Source: three-view drawing plus pictorial views. Frame: mm from the lowest corner of the part. A direction names the side the tool comes from. Round coordinates to 2 decimals unless told otherwise and drop trailing zeros. Order: outer loops, then holes, each group sorted by start corner. A loop starts at its lowest first (then second) coordinate and runs counter-clockwise, first axis right, second up. Notation, with made-up numbers: M 2.25,87.25 L 54.25,87.25 A29 ccw 54.25,120.25 Z; hole C -23,-14 d3. An arc over 180 degrees is marked long. Return JSON: item names as keys, results as strings. Group by question number.
Q1. Ray query, probe 1 along Y at (x, z) = (3.95, 10.5); probe 2 along Z at (x, y) = (5.35, 2.5); probe 3 along Z at (x, y) = (4.8, 9.75). Return the intervals inside material, ascending.
Q2. Cut plane B-B on x = 1.3. Output: boundary loops of the cut face in (y, z).
Q3. Access query for the marked faces 5 and 6. Directions: +Z, -Z, +X, -X, +Y, -Y. A direction counts if a zero-diameter tool reaches every point of the face in a straight line with its end or side. Return the directions, or none.
Q4. Cut plane A-A on y = 2.5. Output: boundary loops of the cut face in (x, z), and give its area (3 significant figures).
Q5. Contact query for a flat-ended pin moving along its axis: pin 1 (3 mm diameter, centred on y = 6.5, z = 6, fed in from -X). Output: stop coordinate, or through.
Q6. Cut plane C-C on z = 15. Output: boundary loops of the cut face in (x, y).
Q7. Mould query, pull axis Z, two halves, no side actions, for the marked faces 1, 2, 3 and 4. Classes: released by +Z, released by -Z, zero draft, split by the parting line, or undercut.
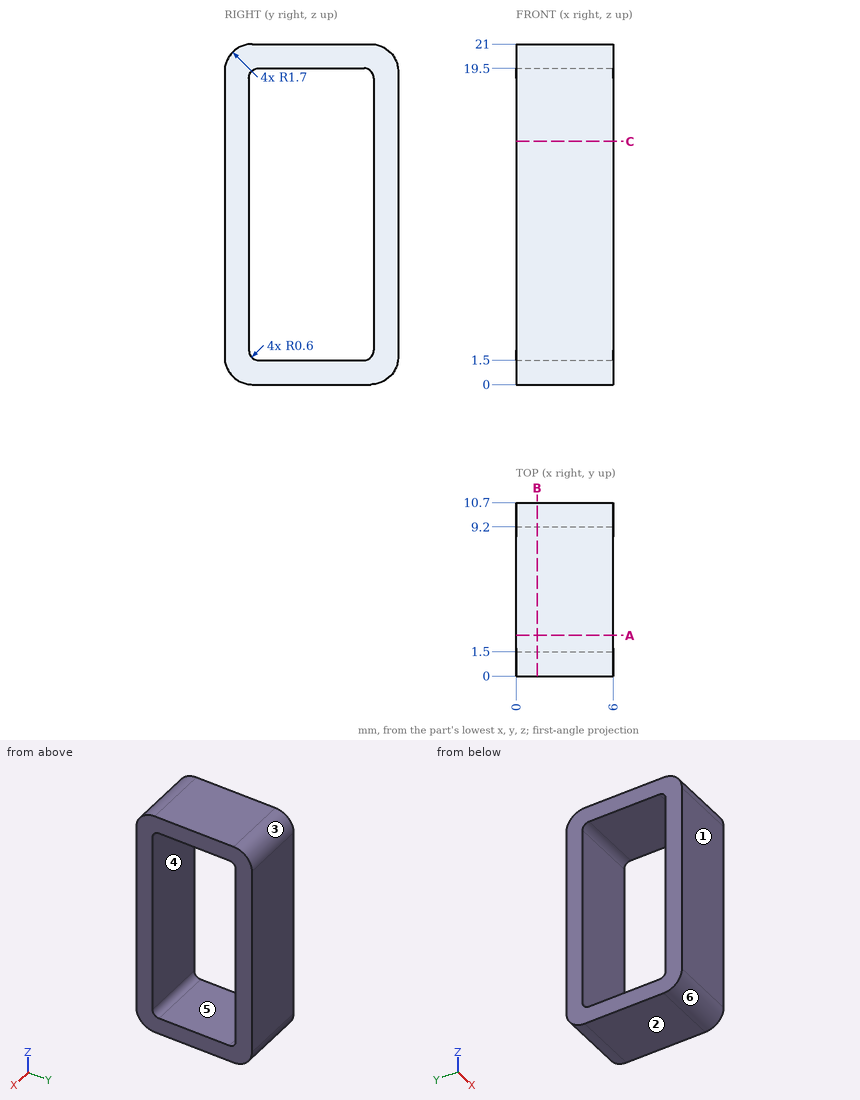
Result sheet:
{
 "1": {"probe 1": "y = 0 to 1.5, 9.2 to 10.7", "probe 2": "z = 0 to 1.5, 19.5 to 21", "probe 3": "z = 0.17 to 20.83"},
 "2": {"outline": "M 0,1.7 A1.7 ccw 1.7,0 L 9,0 A1.7 ccw 10.7,1.7 L 10.7,19.3 A1.7 ccw 9,21 L 1.7,21 A1.7 ccw 0,19.3 Z; hole M 1.5,2.1 A0.6 ccw 2.1,1.5 L 8.6,1.5 A0.6 ccw 9.2,2.1 L 9.2,18.9 A0.6 ccw 8.6,19.5 L 2.1,19.5 A0.6 ccw 1.5,18.9 Z"},
 "3": {"face 5": "+X, -X", "face 6": "-Z, +X, -X, -Y"},
 "4": {"outline": "M 0,0 L 6,0 L 6,1.5 L 0,1.5 Z; M 0,19.5 L 6,19.5 L 6,21 L 0,21 Z", "area": "18.0 mm²"},
 "5": {"pin 1": "passes through"},
 "6": {"outline": "M 0,0 L 6,0 L 6,1.5 L 0,1.5 Z; M 0,9.2 L 6,9.2 L 6,10.7 L 0,10.7 Z"},
 "7": {"face 1": "zero draft", "face 2": "released by -Z", "face 3": "released by +Z", "face 4": "undercut"}
}
